Design review of the part built by this model. Coordinates are the model's own, in mm. A direction names the side the tool comes from. Round coordinates to 2 decimals unless told otherwise and drop trailing zeros. Write each loop counter-clockwise with the first axis right and the second up, starting at its lowest first coordinate (ties: lowest second). Pieces come first, ordered by that corner, then holes. Notation, with made-up numbers: (38.25, 19.5) - (74.25, 19.5) arc R19 cw to (74.25, 41.5) - close; hole circle Ø1 at (-7, 68.5). An arc over 180 degrees is marked (long way). Use one line per item in the form item = value.
```python
from build123d import *

# Parameters (mm, degrees)
BOSS_EXTRUDE1_DEPTH = 6
BOSS_EXTRUDE2_DEPTH = 30


with BuildPart() as part:
    # Sketch1 → Boss-Extrude1 (new body)
    with BuildSketch(Plane(origin=(0, 0, 0), x_dir=(1, 0, 0), z_dir=(0, 1, 0))):
        Polygon((0, 0), (20, 0), (20, 50), (28.859023883, 62.104449423), (14.00827122, 72.973442133), (0, 53.833363868), align=None)
    extrude(amount=BOSS_EXTRUDE1_DEPTH)

    # Sketch2 → Boss-Extrude2 (add)
    with BuildSketch(Plane(origin=(0, 6, 0), x_dir=(1, 0, 0), z_dir=(0, 1, 0))):
        Polygon((14.00827122, 72.973442133), (8.22967873, 65.077913072), (23.080431394, 54.208920362), (28.859023883, 62.104449423), align=None)
    extrude(amount=BOSS_EXTRUDE2_DEPTH)


solid = part.part
```
Q1. Machinability: for faces 1 (the flat face through (11, 6, -33)), 2 (the flat face through (20, 3, -25)), 3 (the flat face through (11, 0, -37)), which of the approach directions +Z, -Z, +X, -X, +Y, -Y give a long, thin tool a straight path to every point of the face, cutting with its end or side? Answer none if there is none.
Calculated:
face_1 = +Z, -X, +Y
face_2 = +Z, +X, +Y, -Y
face_3 = +Z, -Z, +X, -X, -Y
Q2. For P1, Ø10, axis at y = 4.5, z = -14.5, coming from the +X side; P2, Ø4, axis at x = 24.5, y = 27, coming from the +Z side; P3, Ø2, axis at x = 8, y = 25, coming from the +Z side, all flat-tipped, find the tip position at first contact; note any pin that passes through.
Calculated:
P1 = 20
P2 = -54.21
P3 = -64.51
Q3. We need section A-A on x = 9.5. Write out the cut boundary in (y, z).
Calculated:
outline = (0, -66.81) - (36, -66.81) - (36, -64.15) - (6, -64.15) - (6, 0) - (0, 0) - close
Q4. We need section C-C on y = 28. Write out the cut boundary in (x, z).
Calculated:
outline = (8.23, -65.08) - (14.01, -72.97) - (28.86, -62.1) - (23.08, -54.21) - close
Q5. We need section D-D on z = -46.5. Write out the cut boundary in (x, y), then the cut area to 3 significant figures.
Calculated:
outline = (0, 0) - (20, 0) - (20, 6) - (0, 6) - close
area = 120 mm2
Q6. We need section B-B on z = -66.5. Write out the cut boundary in (x, y), then the cut area to 3 significant figures.
Calculated:
outline = (9.27, 0) - (22.85, 0) - (22.85, 36) - (9.27, 36) - close
area = 489 mm2
Q7. To check wall thickness, follow line 1 along Y through (x, z) = (2, -27); line 2 along X through (y, z) = (5, -45.5); line 3 along Z through (x, y) = (6.5, 4.5). State the ranges of each line that lie inside material, in increasing order. Write a range as from..to.
Calculated:
line_1 = 0..6
line_2 = 0..20
line_3 = -62.71..0
